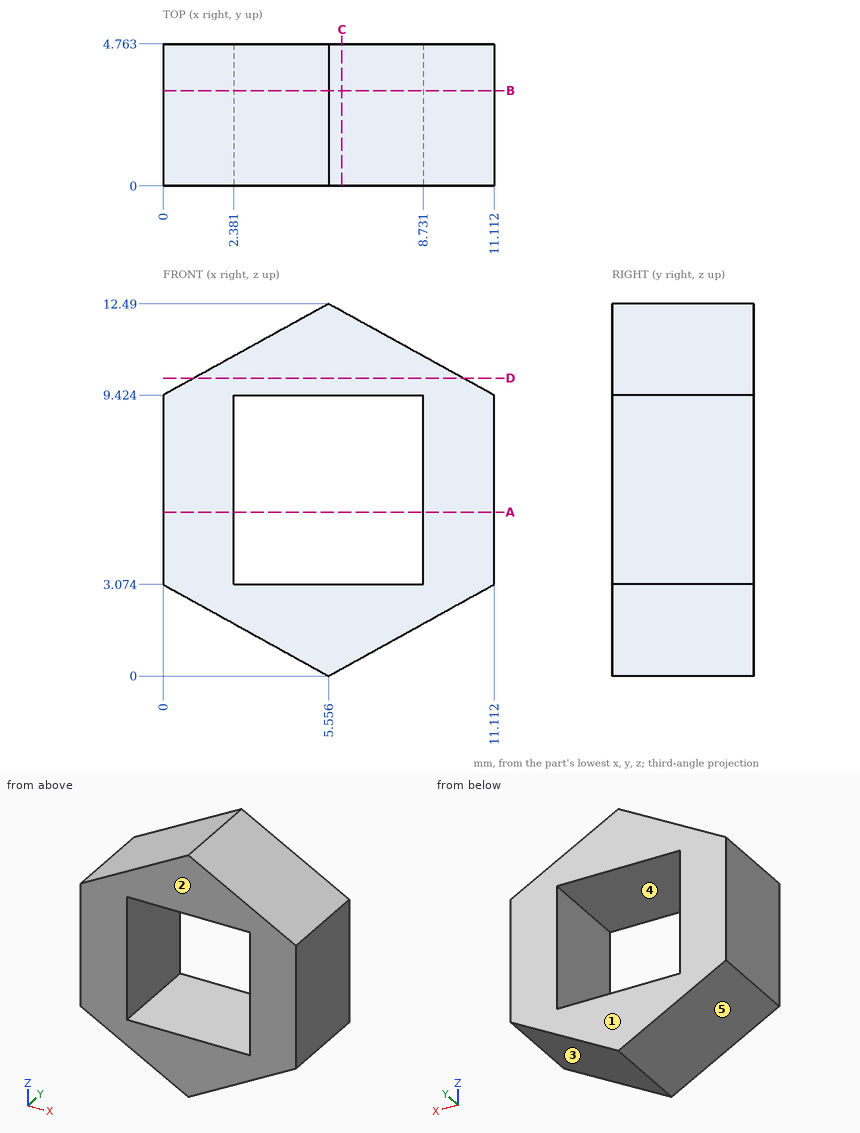
Geometry check sheet. Reference: drawing and pictorial views, mm from the part's lowest x, y, z. A direction names the side the tool comes from. Round coordinates to 2 decimals unless told otherwise and drop trailing zeros. Loops run counter-clockwise (first coordinate to the right, second up) from the corner with the lowest first, then second, coordinate; pieces in that order, holes last. Notation, with made-up numbers: (8.5, 89) - (35.5, 89) arc R33 cw to (35.5, 117) - close; hole circle Ø11 at (31, -15.75). An arc over 180 degrees is marked (long way). Answer in a Markdown table with one row per item. Add a question column.
Q1. Gauge pin test, flat end, axial feed: pin 1 (1.5 mm diameter, centred on x = 2.5, z = 7.5, fed in from -Y). Record the tip position at first contact, or that the pin passes through.
Q2. Release check for a two-part mould opening along Y. For the marked faces 1, 2 and 3 record: pulls with the +Y half, pulls with the -Y half, needs draft (parallel to the pull), parting line crosses it, or undercut.
Q3. Section check C-C on x = 6. Enter the section's corners in (y, z) (1 decimal).
Q4. Tool access check on the marked faces 4 and 5. Record the directions out of +Z, -Z, +X, -X, +Y, -Y that give a thin tool (end or side, any length) a straight path to the whole face; none if there is none.
Q5. Section check A-A on z = 5.5. Enter the section's corners in (x, y), plus the area to 3 significant figures.
Q6. Material ranges on line 1 (X direction, y = 4.5, z = 6); line 2 (Z direction, x = 5, y = 3) (1 decimal); line 3 (Z direction, x = 6, y = 2.2) (1 decimal), recorded low to high.
Q7. Section check D-D on z = 10. Enter the section's corners in (x, y).
Q8. Section check B-B on y = 3.2. Enter the section's corners in (x, z) (1 decimal).
Found:
| question | item | result |
|---|---|---|
| 1 | pin 1 | stops at y = 0 |
| 2 | face 1 | pulls with the +Y half |
| 2 | face 2 | pulls with the -Y half |
| 2 | face 3 | needs draft |
| 3 | outline | (0, 0.2) - (4.8, 0.2) - (4.8, 3.1) - (0, 3.1) - close; (0, 9.4) - (4.8, 9.4) - (4.8, 12.2) - (0, 12.2) - close |
| 4 | face 4 | +Y, -Y |
| 4 | face 5 | -Z, -X, +Y, -Y |
| 5 | outline | (0, 0) - (2.38, 0) - (2.38, 4.76) - (0, 4.76) - close; (8.73, 0) - (11.11, 0) - (11.11, 4.76) - (8.73, 4.76) - close |
| 5 | area | 22.7 mm² |
| 6 | line 1 | x = 0 to 2.38, 8.73 to 11.11 |
| 6 | line 2 | z = 0.3 to 3.1, 9.4 to 12.2 |
| 6 | line 3 | z = 0.2 to 3.1, 9.4 to 12.2 |
| 7 | outline | (1.04, 0) - (10.07, 0) - (10.07, 4.76) - (1.04, 4.76) - close |
| 8 | outline | (0, 3.1) - (5.6, 0) - (11.1, 3.1) - (11.1, 9.4) - (5.6, 12.5) - (0, 9.4) - close; hole (2.4, 3.1) - (8.7, 3.1) - (8.7, 9.4) - (2.4, 9.4) - close |
